Autodesk Inventor part; units mm, degrees
ref_plane "YZ Plane" through (0, 0, 0) normal (1, 0, 0) x (0, 1, 0)
ref_plane "XZ Plane" through (0, 0, 0) normal (0, 1, 0) x (-1, 0, 0)
ref_plane "XY Plane" through (0, 0, 0) normal (0, 0, 1) x (1, 0, 0)
sketch "Sketch1" plane through (0, 0, 0) normal (1, 0, 0) x (0, 1, 0)
  circle A0 centre (0, 0) radius 50
  dimension "d0" = 100
extrude "Extrusion1" add sketch "Sketch1" along normal mid plane 7
sketch "Sketch2" plane through (-3.5, 0, 0) normal (-1, 0, 0) x (0, 0, 1)
  circle A0 centre (0, 0) radius 50
  circle A1 centre (0, 0) radius 47.3
  dimension "d4" = 47.3
extrude "Extrusion2" cut sketch "Sketch2" against normal blind 1.5 contours A1
mirror "Mirror1" about plane through (0, 0, 0) normal (1, 0, 0) of "Extrusion2"
chamfer "Chamfer1" distance 1.61 angle 55 1 edges at (3.5, -50, 0) measured on face at (3.5, 0, -48.0382)
sketch "Sketch3" plane through (-2, 0, 0) normal (-1, 0, 0) x (0, 0, 1)
  circle A0 centre (0, 0) radius 20
  dimension "d10" = 40
extrude "Extrusion3" cut sketch "Sketch3" against normal through all
chamfer "Chamfer2" distance 1.61 angle 55 1 edges at (-3.5, -50, 0) measured on face at (-3.5, 0, -48.0382)
equation "\"d13\" = d7"
properties part number "Clamex grooving Tool" material "Stainless Steel"
Input: part model. Units: mm. Frame: model coordinates. A direction names the side the tool comes from. Round coordinates to 2 decimals unless told otherwise and drop trailing zeros. Write each loop counter-clockwise with the first axis right and the second up, starting at its lowest first coordinate (ties: lowest second). Pieces come first, ordered by that corner, then holes.
1) Contact query for flat-ended pins moving along their axis: P1, Ø2, axis at x = -1.5, y = 28.5, coming from the -Z side; P2, Ø2, axis at y = 29.5, z = 0.5, coming from the +X side; P3, Ø1, axis at x = 1, z = 37.5, coming from the -Y side. Output: stop coordinate, or through.
2) Reachability of faces 4 (the cylindrical face through (0.02, 47.69, 15.02)), 5 (the cylindrical face through (2.76, 46.175, -10.254)), 6 (the flat face through (-2, -20.4, -0.7)) from +Z, -Z, +X, -X, +Y, -Y: full face, straight path, thin tool, end or side. Return the list, or none.
3) Cut plane A-A (z = 0). Return the cut outline in (x, y).
4) Draft query along Y for faces 1 (the flat face through (2, -20.4, 0.7)), 2 (the conical face through (-3.356, -10.512, -47.338)), 3 (the flat face through (-3.5, 10.5, -46.4)). Return one class per face: pulls with the +Y half, pulls with the -Y half, needs draft (parallel to the pull), parting line crosses it, or undercut.
5) Ray query, L1, parallel to X at y = -8, z = -43.5; L2, parallel to Y at x = -2.25, z = -37.5; L3, parallel to Y at x = -1.25, z = 6. Return the intervals inside material, ascending.
Geometry says:
1. P1: stops at z = -41.73
1. P2: stops at x = 2
1. P3: stops at y = -33.63
2. face 4: +X, -X
2. face 5: +X
2. face 6: -X
3. outline: (-3.5, -48.39) - (-1.2, -50) - (1.2, -50) - (3.5, -48.39) - (3.5, -47.3) - (2, -47.3) - (2, -20) - (-2, -20) - (-2, -47.3) - (-3.5, -47.3) - close; (-3.5, 47.3) - (-2, 47.3) - (-2, 20) - (2, 20) - (2, 47.3) - (3.5, 47.3) - (3.5, 48.39) - (1.2, 50) - (-1.2, 50) - (-3.5, 48.39) - close
4. face 1: undercut
4. face 2: parting line crosses it
4. face 3: needs draft
5. L1: x = -2 to 2
5. L2: y = -31.95 to -28.83, 28.83 to 31.95
5. L3: y = -49.6 to -19.08, 19.08 to 49.6
